Source: CAD feature listing. Evaluate the final solid. Frame: model axes, mm. A direction names the side the tool comes from. Round coordinates to 2 decimals unless told otherwise and drop trailing zeros. Write each loop counter-clockwise with the first axis right and the second up, starting at its lowest first coordinate (ties: lowest second). Pieces come first, ordered by that corner, then holes.
Autodesk Inventor part; units mm, degrees
ref_plane "YZ Plane" through (0, 0, 0) normal (1, 0, 0) x (0, 1, 0)
ref_plane "XZ Plane" through (0, 0, 0) normal (0, 1, 0) x (-1, 0, 0)
ref_plane "XY Plane" through (0, 0, 0) normal (0, 0, 1) x (1, 0, 0)
sketch "Szkic8" plane through (0, 0, 0) normal (0, 1, 0) x (-1, 0, 0)
  circle A0 centre (0, 0) radius 35
  circle A1 centre (0, 0) radius 33
  dimension "d53" = 70
  dimension "d54" = 2
extrude "Wyciągnięcie proste2" add sketch "Szkic8" along normal mid plane 160
sketch "Szkic13" plane through (0, 0, 0) normal (0, 0, 1) x (1, 0, 0)
  circle A0 centre (0, 0) radius 14.5
  circle A1 centre (0, 0) radius 12.5
  dimension "d67" = 29
  dimension "d68" = 2
extrude "Wyciągnięcie proste6" add sketch "Szkic13" along normal blind 38.5
sketch "Szkic14" plane through (0, 0, 38.5) normal (0, 0, 1) x (1, 0, 0)
  circle A0 centre (0, 0) radius 12.5
extrude "Wyciągnięcie proste7" cut sketch "Szkic14" against normal blind 38.5
sketch "Szkic15" plane through (0, -80, 0) normal (0, -1, 0) x (1, 0, 0)
  circle A0 centre (0, 0) radius 33
extrude "Wyciągnięcie proste8" cut sketch "Szkic15" against normal blind 160
fillet "Zaokrąglenie3" radius 2 2 edges at (0.0009, 14.5, 35) (-0.0009, -14.5, 35)
fillet "Zaokrąglenie4" radius 4 2 edges at (0.0036, -12.5, 33) (-0.005, 12.5, 33)
equation "\"d53\" = OD"
equation "\"d54\" = THK"
equation "\"d55\" = L1"
equation "\"d67\" = OD2"
equation "\"d68\" = THK"
equation "\"d69\" = L2"
equation "\"d71\" = L2"
equation "\"d73\" = L1"
equation "\"d75\" = THK"
equation "\"d76\" = 2 * THK"
equation "\"SzerokośćGięciaPodcięcia\" = Grubość"
equation "\"RozmiarPodcięciaNarożnika\" = 4 * Grubość"
equation "\"PromieńPrzejścia\" = PromieńGięcia"
equation "\"Rozmiar_promienia_Jacobiego\" = PromieńGięcia"
equation "\"Wielk_odstępu\" = Grubość"
equation "\"d2\" = PromieńGięcia"
equation "\"d23\" = PromieńGięcia"
equation "\"OD\" = 70"
equation "\"THK\" = 2"
equation "\"L1\" = 160"
equation "\"L2\" = 38.5"
equation "\"OD2\" = 29"
properties part number "Trójnik red. krótki  Ø70 29 70 s=2 L=160" material "304"
1) Section query C-C on y = 68.5. Return the cut outline in (x, z), then the cut area to 3 significant figures.
Taken from the geometry:
outline: circle Ø70 at (0, 0); hole circle Ø66 at (0, 0)
area: 427 mm2
2) Section query D-D on x = 0. State how many separate pieces and enclosed holes the cut face has, then the cut area to 3 significant figures.
Taken from the geometry:
separate pieces: 3
enclosed holes: 0
area: 599 mm2
3) Pull-direction query (X, two-part tool) for faces 1 (the face through (7.154, 1.12, -32.215)), 2 (the face through (-11, 7, 38.5)), 3 (the face through (-18.82, -1.12, -29.51)); classes: released by +X, released by -X, zero draft, split by the parting line, or undercut.
Taken from the geometry:
face 1: undercut
face 2: zero draft
face 3: split by the parting line
4) Section query A-A on z = 0. Return the cut outline in (x, y).
Taken from the geometry:
outline: (-35, -80) - (-33, -80) - (-33, 80) - (-35, 80) - close; (33, -80) - (35, -80) - (35, 80) - (33, 80) - close
5) Section query B-B on x = 19.5. Return the cut outline in (y, z).
Taken from the geometry:
outline: (-80, -29.06) - (80, -29.06) - (80, -26.62) - (-80, -26.62) - close; (-80, 26.62) - (80, 26.62) - (80, 29.06) - (-80, 29.06) - close
6) Material intervals for line 1 (Z direction, x = 1, y = -16.5); line 2 (X direction, y = 0, z = 37); line 3 (Z direction, x = 9.5, y = -52.5), sorted ascending.
Taken from the geometry:
line 1: z = -34.99 to -32.98, 32.98 to 34.99
line 2: x = -14.5 to -12.5, 12.5 to 14.5
line 3: z = -33.69 to -31.6, 31.6 to 33.69
7) Contact query for flat-ended pins moving along their axis: P1, Ø2, axis at y = -26, z = -18, coming from the +X side; P2, Ø15, axis at x = 0, y = 0, coming from the -Z side; P3, Ø4, axis at y = -35.5, z = 21.5, coming from the +X side. Output: stop coordinate, or through.
Taken from the geometry:
P1: stops at x = 30.59
P2: stops at z = -35
P3: stops at x = 29.06
8) Reachability of faces 4 (the face through (-12.488, -0.55, 36.368)), 5 (the face through (23.5, 80, 23.5)) from +Z, -Z, +X, -X, +Y, -Y: full face, straight path, thin tool, end or side. Return the list, or none.
Taken from the geometry:
face 4: +Z
face 5: +Z, -Z, +X, -X, +Y
